Can you work these out from the drawing? Everything is in mm from the part's minimum corner. A direction names the side the tool comes from. Round coordinates to 2 decimals unless told otherwise and drop trailing zeros. Write each loop counter-clockwise with the first axis right and the second up, starting at its lowest first coordinate (ties: lowest second). Pieces come first, ordered by that corner, then holes. Notation, with made-up numbers: (85, 25.25) -> (115, 25.25) arc R25 ccw to (115, 61.25) -> close; hole circle Ø8 at (83.25, 70). An arc over 180 degrees is marked (long way). Answer as CSV lines item,"result". Start each with the question number.
Q1. Will these pins go through, and if not, where does the flat tip stop? pin 1 Ø3 at (x, y) = (3.5, 5.5) entering from +Z; pin 2 Ø3.5 at (x, y) = (12, 11.5) entering from -Z; pin 3 Ø1.4 at (x, y) = (11, 3) entering from +Z (3 decimals).
Q2. For the marked faces 5 and 6, which set-ups out of +Z, -Z, +X, -X, +Y, -Y let a thin tool reach every point of the face, with its end or its side?
Q3. If I drill on line 1 (Y direction, x = 11, z = 0.75); line 2 (Y direction, x = 11, z = 1.4); line 3 (Y direction, x = 11, z = 2.1), over which ranges is the centre line in solid material (lowest first)? Write a range as [from, to].
Q4. If we mould it in two halves opening along Y, with no side actions, what happens to the marked faces 1, 2, 3 and 4? For each: pulls with the +Y half, pulls with the -Y half, needs draft (parallel to the pull), parting line crosses it, or undercut.
Q5. Imagine slicing it at D-D on y = 9.5. Please give me the cut outline in (x, z).
Q6. Imagine slicing it at C-C on x = 11. Please give me the cut outline in (y, z), and give its area (3 significant figures).
Q7. Imagine slicing it at A-A on z = 1.3. Please give me the cut outline in (x, y).
Q8. Imagine slicing it at B-B on x = 3.25. Please give me the cut outline in (y, z), and give its area (3 significant figures).
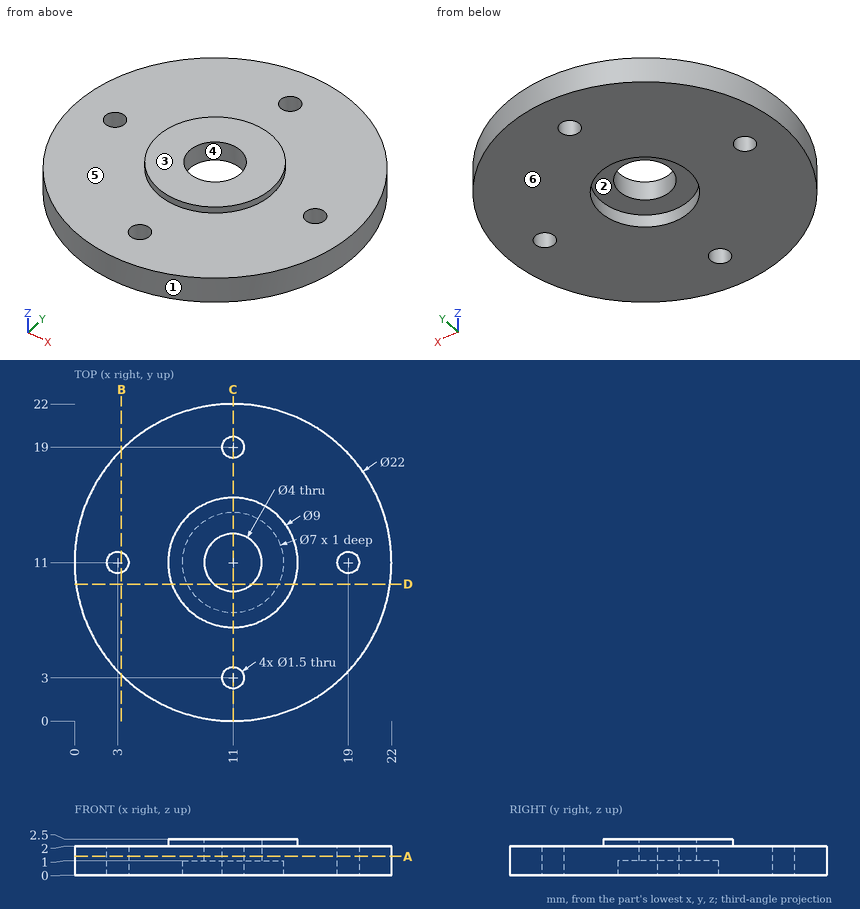
Checks:
1,pin 1,"z = 2"
1,pin 2,"z = 1"
1,pin 3,"through"
2,face 5,"+Z"
2,face 6,"-Z, +X, -X, +Y, -Y"
3,line 1,"[0, 2.25], [3.75, 7.5], [14.5, 18.25], [19.75, 22]"
3,line 2,"[0, 2.25], [3.75, 9], [13, 18.25], [19.75, 22]"
3,line 3,"[6.5, 9], [13, 15.5]"
4,face 1,"parting line crosses it"
4,face 2,"undercut"
4,face 3,"needs draft"
4,face 4,"undercut"
5,outline,"(0.1, 0) -> (7.84, 0) -> (7.84, 1) -> (9.68, 1) -> (9.68, 2.5) -> (6.76, 2.5) -> (6.76, 2) -> (0.1, 2) -> close; (12.32, 1) -> (14.16, 1) -> (14.16, 0) -> (21.9, 0) -> (21.9, 2) -> (15.24, 2) -> (15.24, 2.5) -> (12.32, 2.5) -> close"
6,outline,"(0, 0) -> (2.25, 0) -> (2.25, 2) -> (0, 2) -> close; (3.75, 0) -> (7.5, 0) -> (7.5, 1) -> (9, 1) -> (9, 2.5) -> (6.5, 2.5) -> (6.5, 2) -> (3.75, 2) -> close; (13, 1) -> (14.5, 1) -> (14.5, 0) -> (18.25, 0) -> (18.25, 2) -> (15.5, 2) -> (15.5, 2.5) -> (13, 2.5) -> close; (19.75, 0) -> (22, 0) -> (22, 2) -> (19.75, 2) -> close"
6,area,"29.5 mm^2"
7,outline,"circle Ø22 at (11, 11); hole circle Ø1.5 at (3, 11); hole circle Ø4 at (11, 11); hole circle Ø1.5 at (11, 3); hole circle Ø1.5 at (11, 19); hole circle Ø1.5 at (19, 11)"
8,outline,"(3.19, 0) -> (10.29, 0) -> (10.29, 2) -> (3.19, 2) -> close; (11.71, 0) -> (18.81, 0) -> (18.81, 2) -> (11.71, 2) -> close"
8,area,"28.4 mm^2"
